Check sheet for the modelled part. Datum: model origin and axes. Units: mm. A direction names the side the tool comes from. Give positions to 0.01 mm unless a question says otherwise; leave off trailing zeros. Order: outer loops, then holes, each group sorted by start corner. A loop starts at its lowest first (then second) coordinate and runs counter-clockwise, first axis right, second up.
```python
from build123d import *

# Parameters (mm, degrees)
EXTRUDE_1_DEPTH      = 14
CUT_EXTRUDE_1_DEPTH  = 44
SKETCH_3_W           = 6.2
SKETCH_3_H           = 6.2
CUT_EXTRUDE_2_DEPTH  = 4
SKETCH_4_R           = 4
CUT_EXTRUDE_3_DEPTH  = 5
SKETCH_5_R           = 2.6
CUT_EXTRUDE_4_DEPTH  = 5
SKETCH_6_R           = 4
EXTRUDE_2_DEPTH      = 10
SKETCH_7_W           = 6.2
SKETCH_7_H           = 4
EXTRUDE_3_DEPTH      = 40
CUT_EXTRUDE_5_DEPTH  = 50
SKETCH_9_W           = 20
SKETCH_9_H           = 25
EXTRUDE_4_DEPTH      = 44
CUT_EXTRUDE_6_DEPTH  = 44
EXTRUDE_5_DEPTH      = 44
SKETCH_12_W          = 6.9
SKETCH_12_H          = 22.5
CUT_EXTRUDE_7_DEPTH  = 50
SKETCH_13_R          = 3.5
CUT_EXTRUDE_9_DEPTH  = 3
CUT_EXTRUDE_START    = -3
SKETCH_14_R          = 3.5
CUT_EXTRUDE_10_DEPTH = 3
SKETCH_15_R          = 1.51
CUT_EXTRUDE_11_DEPTH = 200


with BuildPart() as part:
    # 草图1 → 凸台-拉伸1 (new body)
    with BuildSketch(Plane.XY):
        Polygon((-15, 22), (-15, -22), (15, -22), (15, 22), (0, 22), align=None)
    extrude(amount=EXTRUDE_1_DEPTH)

    # 草图2 → 切除-拉伸1 (cut)
    with BuildSketch(Plane(origin=(0, 22, 0), x_dir=(1, 0, 0), z_dir=(0, 1, 0))):
        Polygon((-15, 0), (-15, -14), (-10, -4), (-3.1, -4), (-3.1, 0), align=None)
        Polygon((3.1, -4), (10, -4), (15, -14), (15, 0), (3.1, 0), align=None)
    extrude(amount=-CUT_EXTRUDE_1_DEPTH, mode=Mode.SUBTRACT)

    # 草图3 → 切除-拉伸2 (cut)
    with BuildSketch(Plane(origin=(0, 0, 0), x_dir=(-1, 0, 0), z_dir=(0, 0, -1))):
        Rectangle(SKETCH_3_W, SKETCH_3_H)
    extrude(amount=-CUT_EXTRUDE_2_DEPTH, mode=Mode.SUBTRACT)

    # 草图4 → 切除-拉伸3 (cut)
    with BuildSketch(Plane.XY.offset(14)):
        Circle(SKETCH_4_R)
    extrude(amount=-CUT_EXTRUDE_3_DEPTH, mode=Mode.SUBTRACT)

    # 草图5 → 切除-拉伸4 (cut)
    with BuildSketch(Plane.XY.offset(9)):
        Circle(SKETCH_5_R)
    extrude(amount=-CUT_EXTRUDE_4_DEPTH, mode=Mode.SUBTRACT)

    # 草图6 → 凸台-拉伸2 (add)
    with BuildSketch(Plane.XY.offset(14)):
        Circle(SKETCH_6_R)
    extrude(amount=-EXTRUDE_2_DEPTH)

    # 草图7 → 凸台-拉伸3 (add)
    with BuildSketch(Plane(origin=(0, -22, 0), x_dir=(-1, 0, 0), z_dir=(0, -1, 0))):
        with Locations((0, -2)):
            Rectangle(SKETCH_7_W, SKETCH_7_H)
    extrude(amount=-EXTRUDE_3_DEPTH)

    # 草图8 → 切除-拉伸5 (cut)
    with BuildSketch(Plane.XZ.offset(22)):
        Polygon((-15, 14), (-10, 4), (-10, 14), align=None)
        Polygon((15, 14), (10, 14), (10, 4), align=None)
    extrude(amount=-CUT_EXTRUDE_5_DEPTH, mode=Mode.SUBTRACT)

    # 草图9 → 凸台-拉伸4 (add)
    with BuildSketch(Plane.XZ.offset(22)):
        with Locations((0, 16.5)):
            Rectangle(SKETCH_9_W, SKETCH_9_H)
    extrude(amount=-EXTRUDE_4_DEPTH)

    # 草图10 → 切除-拉伸6 (cut)
    with BuildSketch(Plane.XZ.offset(22)):
        with BuildLine():
            Line((-10, 29), (-10, 19))
            ThreePointArc((-10, 19), (-7.071067812, 26.071067812), (0, 29))
            Line((0, 29), (-10, 29))
        make_face()
    extrude(amount=-CUT_EXTRUDE_6_DEPTH, mode=Mode.SUBTRACT)

    # 草图11 → 凸台-拉伸5 (add)
    with BuildSketch(Plane.XZ.offset(22)):
        with BuildLine():
            Line((120, 0), (123.1, 0))
            Line((123.1, 0), (123.1, 4))
            Line((123.1, 4), (130, 4))
            Line((130, 4), (130, 19))
            ThreePointArc((130, 19), (127.071067812, 26.071067812), (120, 29))
            Line((120, 29), (110, 29))
            Line((110, 29), (10, 29))
            Line((10, 29), (10, 26.5))
            Line((10, 26.5), (110, 26.5))
            Line((110, 26.5), (110, 4))
            Line((110, 4), (116.9, 4))
            Line((116.9, 4), (116.9, 0))
            Line((116.9, 0), (120, 0))
        make_face()
    extrude(amount=-EXTRUDE_5_DEPTH)

    # 草图12 → 切除-拉伸7 (cut)
    with BuildSketch(Plane(origin=(0, 22, 0), x_dir=(1, 0, 0), z_dir=(0, 1, 0))):
        with Locations((6.55, -15.25)):
            Rectangle(SKETCH_12_W, SKETCH_12_H)
        with Locations((113.45, -15.25)):
            Rectangle(SKETCH_12_W, SKETCH_12_H)
    extrude(amount=-CUT_EXTRUDE_7_DEPTH, mode=Mode.SUBTRACT)

    # 草图13 → 切除-拉伸9 (cut)
    with BuildSketch(Plane(origin=(130, 0, 0), x_dir=(0, 0, -1), z_dir=(1, 0, 0))):
        with Locations((-15.4, 0)):
            Circle(SKETCH_13_R)
    extrude(amount=-CUT_EXTRUDE_9_DEPTH, mode=Mode.SUBTRACT)

    # 草图14 → 切除-拉伸10 (cut)
    with BuildSketch(Plane.ZY.offset(10).offset(CUT_EXTRUDE_START)):
        with Locations(Location((15.4, 0, 0), (0, 0, 180))):
            Circle(SKETCH_14_R)
    extrude(amount=CUT_EXTRUDE_10_DEPTH, mode=Mode.SUBTRACT)

    # 草图15 → 切除-拉伸11 (cut)
    with BuildSketch(Plane.ZY.offset(7)):
        with Locations(Location((15.4, 0, 0), (0, 0, 270))):
            Circle(SKETCH_15_R)
    extrude(amount=-CUT_EXTRUDE_11_DEPTH, mode=Mode.SUBTRACT)


solid = part.part
```
(1) Cross-section at D-D on y = -10. Enter the section's corners in (x, z), then the cut area to 3 significant figures.
Response values:
outline: (-10, 4) - (-3.1, 4) - (-3.1, 0) - (3.1, 0) - (3.1, 26.5) - (116.9, 26.5) - (116.9, 0) - (123.1, 0) - (123.1, 4) - (130, 4) - (130, 19) arc R10 ccw to (120, 29) - (0, 29) arc R10 ccw to (-10, 19) - close
area: 946 mm2
(2) Release check for a two-part mould opening along Z. For faces 4 (the face through (-7, 0, 4)), 5 (the face through (127, -2, 15)), 6 (the face through (130, 0, 11)) record: released by +Z, released by -Z, zero draft, split by the parting line, or undercut.
Response values:
face 4: released by -Z
face 5: undercut
face 6: zero draft
(3) Cross-section at C-C on y = 0. Count the separate pieces of the cut face and the enclosed holes in it, then the cut area to 3 significant figures.
Response values:
separate pieces: 3
enclosed holes: 0
area: 843 mm2
(4) Gauge pin test, flat ends, axial feed: pin 1 Ø7.5 at (y, z) = (1, 14) entering from +X; pin 2 Ø5 at (y, z) = (0, 15.4) entering from -X; pin 3 Ø2 at (y, z) = (2, 2) entering from +X; pin 4 Ø5.5 at (x, y) = (-7, -9.5) entering from -Z. Record the tip position at first contact, or that the pin passes through.
Response values:
pin 1: stops at x = 130
pin 2: stops at x = -7
pin 3: stops at x = 123.1
pin 4: stops at z = 4
(5) Cross-section at A-A on z = 6.25. Enter the section's corners in (x, y), then the cut area to 3 significant figures.
Response values:
outline: (-10, -22) - (3.1, -22) - (3.1, 22) - (-10, 22) - close; (116.9, -22) - (130, -22) - (130, 22) - (116.9, 22) - close
area: 1,150 mm2
(6) Material ranges on L1, parallel to X at y = 4, z = 14; L2, parallel to Y at x = -8.95, z = 15.4; L3, parallel to X at y = 14, z = 3, recorded low to high.
Response values:
L1: x = -10 to 3.1, 116.9 to 130
L2: y = -22 to -3.5, 3.5 to 22
L3: x = -3.1 to 3.1, 116.9 to 123.1
(7) Cross-section at B-B on z = 15.4. Enter the section's corners in (x, y).
Response values:
outline: (-10, -22) - (3.1, -22) - (3.1, -1.51) - (-7, -1.51) - (-7, -3.5) - (-10, -3.5) - close; (-10, 3.5) - (-7, 3.5) - (-7, 1.51) - (3.1, 1.51) - (3.1, 22) - (-10, 22) - close; (116.9, -22) - (130, -22) - (130, -3.5) - (127, -3.5) - (127, -1.51) - (116.9, -1.51) - close; (116.9, 1.51) - (127, 1.51) - (127, 3.5) - (130, 3.5) - (130, 22) - (116.9, 22) - close
(8) Set-up check for faces 1 (the face through (127, 0, 4)), 2 (the face through (-7, 2, 15)), 3 (the face through (59, 0, 26.5)): record each of +Z, -Z, +X, -X, +Y, -Y from which the full face is reachable in a straight line by a thin tool's end or side.
Response values:
face 1: -Z, +X, +Y, -Y
face 2: -X
face 3: -Z, +Y, -Y
